Geometry check sheet. Reference: drawing and pictorial views, mm from the part's lowest x, y, z. A direction names the side the tool comes from. Give positions to 0.01 mm unless a question says otherwise; leave off trailing zeros. Loops run counter-clockwise (first coordinate to the right, second up) from the corner with the lowest first, then second, coordinate; pieces in that order, holes last. Notation, with made-up numbers: M -26,86 L -10,86 A16 ccw -10,107 Z; hole C 50,9 d9. An arc over 180 degrees is marked long. Use CSV: the item, a comma, the result in double quotes.
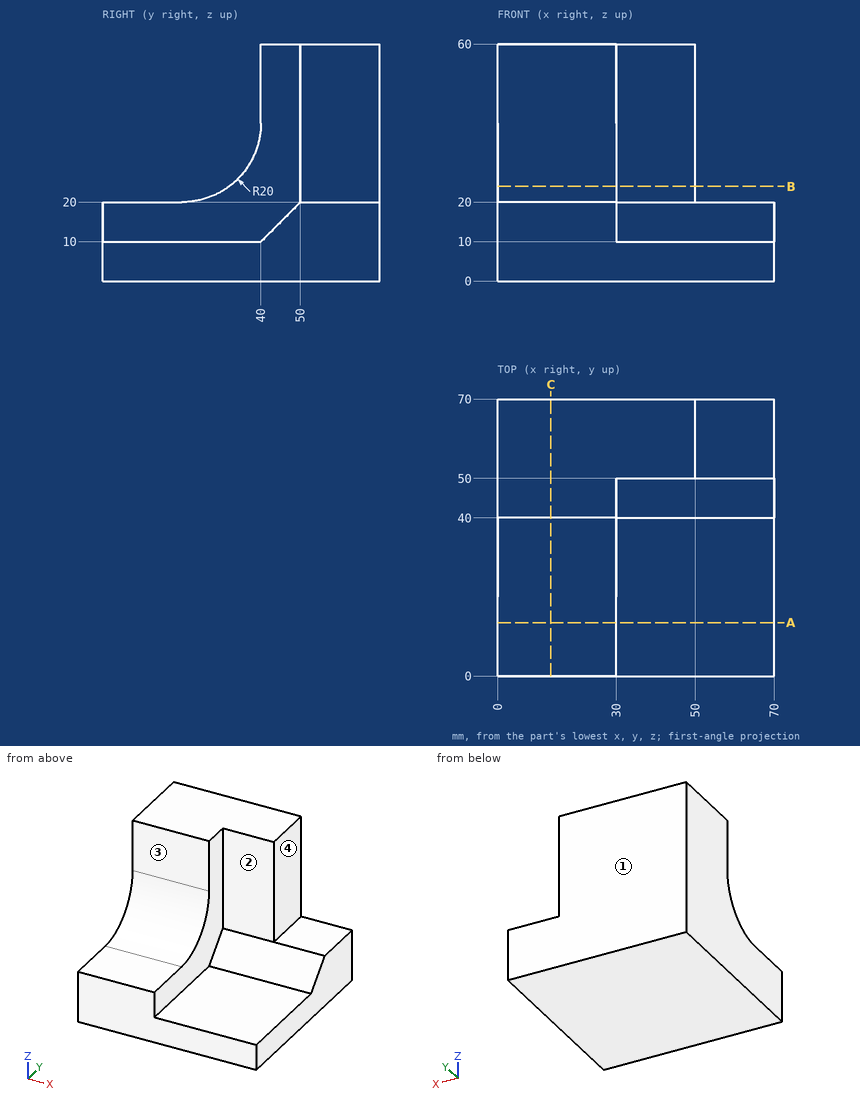
(1) Section check B-B on z = 24. Record the cut outline in (x, y), plus the area to 3 significant figures.
Calculated:
outline,"M 0,32 L 30,32 L 30,50 L 50,50 L 50,70 L 0,70 Z"
area,"1,540 mm²"
(2) Depth check by flat-ended pin: pin 1 Ø4 at (y, z) = (42.5, 17.5) entering from +X; pin 2 Ø10 at (x, y) = (11.5, 6.5) entering from +Z; pin 3 Ø6 at (x, z) = (39.5, 30) entering from -Y. Enter the tip coordinate at first touch or a pass-through.
Calculated:
pin 1,"stops at x = 30"
pin 2,"stops at z = 20"
pin 3,"stops at y = 50"
(3) Scan lines: L1, parallel to Y at x = 20, z = 45; L2, parallel to X at y = 24, z = 13.5; L3, parallel to Y at x = 39.5, z = 37. Record each from-to range of solid material in increasing order. Write a range as from..to.
Calculated:
L1,"y = 40..70"
L2,"x = 0..30"
L3,"y = 50..70"
(4) Section check C-C on x = 13.5. Record the cut outline in (y, z).
Calculated:
outline,"M 0,0 L 70,0 L 70,60 L 40,60 L 40,40 A20 cw 20,20 L 0,20 Z"
(5) Section check A-A on y = 13.5. Record the cut outline in (x, z), plus the area to 3 significant figures.
Calculated:
outline,"M 0,0 L 70,0 L 70,10 L 30,10 L 30,20 L 0,20 Z"
area,"1,000 mm²"
(6) Tool access check on the marked faces 1, 2, 3 and 4. Record the directions out of +Z, -Z, +X, -X, +Y, -Y that give a thin tool (end or side, any length) a straight path to the whole face; none if there is none.
Calculated:
face 1,"+Z, -Z, +X, -X, +Y"
face 2,"+Z, +X, -Y"
face 3,"+Z, +X, -X, -Y"
face 4,"+Z, +X, +Y, -Y"
